Check sheet for the modelled part. Datum: model origin and axes. Units: mm. Face numbers are marked on the shaded views. A direction names the side the tool comes from. Give positions to 0.01 mm unless a question says otherwise; leave off trailing zeros. Order: outer loops, then holes, each group sorted by start corner. A loop starts at its lowest first (then second) coordinate and runs counter-clockwise, first axis right, second up. Notation, with made-up numbers: (33, 2) -> (64, 2) arc R14 cw to (64, 25) -> close; hole circle Ø9 at (89.25, 70.5). An arc over 180 degrees is marked (long way). One line per question, with ' | ' between items.
```python
from build123d import *

# Parameters (mm, degrees)
F0_W     = 60
F0_H     = 25
F1_DEPTH = 20
F2_W     = 21
F2_H     = 17.5
F3_DEPTH = 25.001
F4_R     = 1
F5_SIZE  = 0.5


with BuildPart() as f1:
    # F0 (on Top) → F1 (new body)
    with BuildSketch(Plane.XY):
        Rectangle(F0_W, F0_H)
    extrude(amount=F1_DEPTH)

    # F2 (on face) → F3 (cut, through all)
    with BuildSketch(Plane.XZ.offset(12.5)):
        with Locations((0, 11.25)):
            Rectangle(F2_W, F2_H)
        Polygon((-30, 2.5), (-13, 20), (-30, 20), align=None)
        Polygon((30, 2.5), (30, 20), (13, 20), align=None)
    extrude(amount=-F3_DEPTH, mode=Mode.SUBTRACT)

    # F4
    f4_edges = [f1.edges().sort_by_distance(p)[0] for p in [
        (-10.5, 0, 2.5),
        (10.5, 0, 2.5),
        (-30, 0, 2.5),
        (30, 0, 2.5),
    ]]
    fillet(f4_edges, radius=F4_R)

    # F5
    f5_edges = [f1.edges().sort_by_distance(p)[0] for p in [
        (0, -12.5, 0),
        (30, 0, 0),
        (0, 12.5, 0),
        (-30, 0, 0),
        (-10.5, 0, 20),
        (10.5, 0, 20),
        (30, -12.5, 1.047125),
        (29.926628, -12.5, 2.470229),
        (21.35864, -12.5, 11.395518),
        (-30, -12.5, 1.047125),
        (11.75, -12.5, 20),
        (-29.926628, -12.5, 2.470229),
        (10.5, -12.5, 11.75),
        (-21.35864, -12.5, 11.395518),
        (10.207107, -12.5, 2.792893),
        (-11.75, -12.5, 20),
        (0, -12.5, 2.5),
        (-10.5, -12.5, 11.75),
        (-10.207107, -12.5, 2.792893),
        (-30, 12.5, 1.047125),
        (-29.926628, 12.5, 2.470229),
        (-21.35864, 12.5, 11.395518),
        (30, 12.5, 1.047125),
        (-11.75, 12.5, 20),
        (29.926628, 12.5, 2.470229),
        (-10.5, 12.5, 11.75),
        (21.35864, 12.5, 11.395518),
        (-10.207107, 12.5, 2.792893),
        (11.75, 12.5, 20),
        (0, 12.5, 2.5),
        (10.5, 12.5, 11.75),
        (10.207107, 12.5, 2.792893),
    ]]
    chamfer(f5_edges, length=F5_SIZE)


solid = f1.part
```
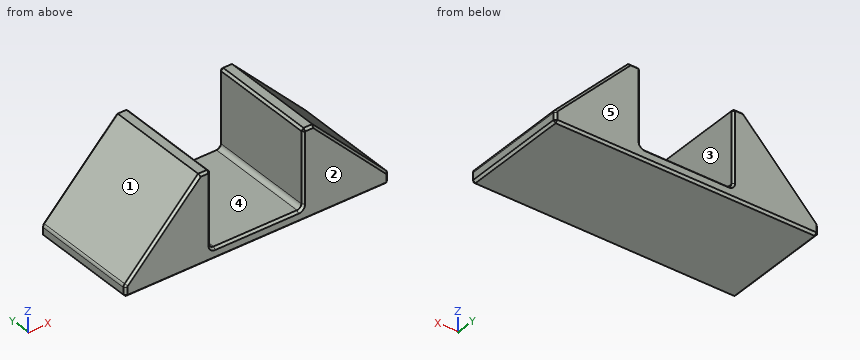
Q1. Section check C-C (x = -8.5). Enter the section's corners in (y, z).
Result sheet:
outline: (-12.5, 0.5) -> (-12, 0) -> (12, 0) -> (12.5, 0.5) -> (12.5, 2) -> (12, 2.5) -> (-12, 2.5) -> (-12.5, 2) -> close
Q2. Section check D-D (z = 18). Enter the section's corners in (x, y), and give its area (3 significant figures).
Result sheet:
outline: (-14.94, -12) -> (-14.25, -12.5) -> (-11, -12.5) -> (-10.5, -12) -> (-10.5, 12) -> (-11, 12.5) -> (-14.25, 12.5) -> (-14.94, 12) -> close; (10.5, -12) -> (11, -12.5) -> (14.25, -12.5) -> (14.94, -12) -> (14.94, 12) -> (14.25, 12.5) -> (11, 12.5) -> (10.5, 12) -> close | area: 221 mm2
Q3. Access from +Z, -Z, +X, -X, +Y, -Y to the whole of each face (thin tool, end or side, straight path). Record for the marked faces 4 and 5.
Result sheet:
face 4: +Z, +Y, -Y | face 5: +Z, -Z, +X, -X, +Y
Q4. Thickness scan on line 1 (X direction, y = 0.5, z = 14.5); line 2 (Z direction, x = -2, y = -1.5); line 3 (X direction, y = -4.75, z = 5.5). Record the ranges inside material, lowest first.
Result sheet:
line 1: x = -18.34 to -10.5, 10.5 to 18.34 | line 2: z = 0 to 2.5 | line 3: x = -27.09 to -10.5, 10.5 to 27.09
Q5. Section check A-A (z = 6.25). Enter the section's corners in (x, y), and give its area (3 significant figures).
Result sheet:
outline: (-26.36, -12) -> (-25.66, -12.5) -> (-11, -12.5) -> (-10.5, -12) -> (-10.5, 12) -> (-11, 12.5) -> (-25.66, 12.5) -> (-26.36, 12) -> close; (10.5, -12) -> (11, -12.5) -> (25.66, -12.5) -> (26.36, -12) -> (26.36, 12) -> (25.66, 12.5) -> (11, 12.5) -> (10.5, 12) -> close | area: 792 mm2
Q6. Mould release check, pull along X, two halves, no side actions. Record for the marked faces 1, 2 and 3: pulls with the +X half, pulls with the -X half, needs draft (parallel to the pull), parting line crosses it, or undercut.
Result sheet:
face 1: pulls with the -X half | face 2: needs draft | face 3: undercut
Q7. Depth check by flat-ended pin: pin 1 Ø6 at (y, z) = (-5.5, 10) entering from +X; pin 2 Ø5.5 at (x, y) = (-1.5, 6) entering from +Z; pin 3 Ø1 at (y, z) = (2, 9) entering from -X. Enter the tip coordinate at first touch or a pass-through.
Result sheet:
pin 1: stops at x = 25.63 | pin 2: stops at z = 2.5 | pin 3: stops at x = -24.17
Q8. Section check B-B (y = -8.5). Enter the section's corners in (x, z).
Result sheet:
outline: (-30, 0.5) -> (-29.5, 0) -> (29.5, 0) -> (30, 0.5) -> (30, 2.09) arc R1 ccw to (29.72, 2.79) -> (13, 20) -> (11, 20) -> (10.5, 19.5) -> (10.5, 3.5) arc R1 cw to (9.5, 2.5) -> (-9.5, 2.5) arc R1 cw to (-10.5, 3.5) -> (-10.5, 19.5) -> (-11, 20) -> (-13, 20) -> (-29.72, 2.79) arc R1 ccw to (-30, 2.09) -> close
